from build123d import *

# Parameters (mm, degrees)
BOSS_EXTRUDE1_DEPTH   = 50
SKETCH4_R             = 3
BOSS_EXTRUDE2_DEPTH   = 5
M4X0_7_TAPPED_HOLE1_D = 3.3
FILLET1_R             = 0.5


with BuildPart() as part:
    # Sketch1 → Boss-Extrude1 (new body)
    with BuildSketch(Plane.XY):
        Polygon((0, 0), (0, 4.5), (6.75, 4.5), (6.75, 6.75), (27.25, 6.75), (27.25, 4.5), (34, 4.5), (34, 0), (23.25, 0), (23.25, 3.75), (10.75, 3.75), (10.75, 0), align=None)
    extrude(amount=BOSS_EXTRUDE1_DEPTH)

    # Sketch4 → Boss-Extrude2 (add)
    with BuildSketch(Plane(origin=(0, 6.75, 0), x_dir=(1, 0, 0), z_dir=(0, 1, 0))):
        with Locations(Location((17, -15, 0), (0, 0, 90))):
            Circle(SKETCH4_R)
        with Locations(Location((17, -35, 0), (0, 0, 90))):
            Circle(SKETCH4_R)
    extrude(amount=BOSS_EXTRUDE2_DEPTH)

    # M4x0.7 Tapped Hole1 (through all)
    with Locations(Plane(origin=(17, 11.75, 15), x_dir=(0, 0, 1), z_dir=(0, 1, 0))):
        with Locations((0, 0), (20, 0)):
            Hole(M4X0_7_TAPPED_HOLE1_D / 2)

    # Fillet1
    fillet1_edges = [part.edges().sort_by_distance(p)[0] for p in [
        (17, 11.75, 18),
        (17, 11.75, 38),
    ]]
    fillet(fillet1_edges, radius=FILLET1_R)


solid = part.part
Input: part model. Units: mm. Frame: model coordinates. A direction names the side the tool comes from. Coordinates: 2 decimals unless noted, no trailing zeros. Loops run counter-clockwise (first coordinate to the right, second up) from the corner with the lowest first, then second, coordinate; pieces in that order, holes last.
(1) Material intervals for probe 1 along X at (y, z) = (6.25, 15); probe 2 along Y at (x, z) = (32, 14.5); probe 3 along X at (y, z) = (0.75, 43.5), sorted ascending.
(2) Set-up query: faces 1 (the face through (10.75, 2, 25)), 2 (the face through (17, 9, 38)), 3 (the face through (31, 4.5, 25)). Return all of +Z, -Z, +X, -X, +Y, -Y with unobstructed straight access to the full face (end or side cutting, diameter ignored); none if empty.
(3) Section B-B on x = 17. Return the cut outline in (y, z).
(4) Section D-D on y = 9.75. Return the cut outline in (x, z).
(5) Pull-direction query (Z, two-part tool) for faces 4 (the face through (18.8, 9, 17.4)), 5 (the face through (17, 4, 0)), 6 (the face through (5, 0, 25)); classes: released by +Z, released by -Z, zero draft, split by the parting line, or undercut.
(6) Section A-A on z = 15. Return the cut outline in (x, y).
(7) Section C-C on y = 1.5. Return the cut outline in (x, z), then the cut area to 4 significant figures.
(8) First-contact query: pin 1 Ø5 at (x, z) = (8.5, 9) entering from +Y; pin 2 Ø4.5 at (x, z) = (17, 15) entering from -Y; pin 3 Ø1.1 at (y, z) = (6, 30.5) entering from +X. Flat tips, straight axial feed; report the tip coordinate or a pass-through.
Data:
1. probe 1: x = 6.75 to 15.35, 18.65 to 27.25
1. probe 2: y = 0 to 4.5
1. probe 3: x = 0 to 10.75, 23.25 to 34
2. face 1: +Z, -Z, -Y
2. face 2: +Y
2. face 3: +Z, -Z, +X, +Y
3. outline: (3.75, 0) - (6.75, 0) - (6.75, 12) - (11.25, 12) arc R0.5 ccw to (11.75, 12.5) - (11.75, 13.35) - (3.75, 13.35) - close; (3.75, 16.65) - (11.75, 16.65) - (11.75, 17.5) arc R0.5 ccw to (11.25, 18) - (6.75, 18) - (6.75, 32) - (11.25, 32) arc R0.5 ccw to (11.75, 32.5) - (11.75, 33.35) - (3.75, 33.35) - close; (3.75, 36.65) - (11.75, 36.65) - (11.75, 37.5) arc R0.5 ccw to (11.25, 38) - (6.75, 38) - (6.75, 50) - (3.75, 50) - close
4. outline: circle Ø6 at (17, 15); circle Ø6 at (17, 35); hole circle Ø3.3 at (17, 15); hole circle Ø3.3 at (17, 35)
5. face 4: undercut
5. face 5: released by -Z
5. face 6: zero draft
6. outline: (0, 0) - (10.75, 0) - (10.75, 3.75) - (15.35, 3.75) - (15.35, 11.75) - (14.5, 11.75) arc R0.5 ccw to (14, 11.25) - (14, 6.75) - (6.75, 6.75) - (6.75, 4.5) - (0, 4.5) - close; (18.65, 3.75) - (23.25, 3.75) - (23.25, 0) - (34, 0) - (34, 4.5) - (27.25, 4.5) - (27.25, 6.75) - (20, 6.75) - (20, 11.25) arc R0.5 ccw to (19.5, 11.75) - (18.65, 11.75) - close
7. outline: (0, 0) - (10.75, 0) - (10.75, 50) - (0, 50) - close; (23.25, 0) - (34, 0) - (34, 50) - (23.25, 50) - close
7. area: 1,075 mm2
8. pin 1: stops at y = 6.75
8. pin 2: stops at y = 3.75
8. pin 3: stops at x = 27.25
